The figure shows three views and two pictorial views of one solid part (mm, origin at its lowest corner). Answer the questions. A direction names the side the tool comes from. Round coordinates to 2 decimals unless told otherwise and drop trailing zeros. Write each loop counter-clockwise with the first axis right and the second up, starting at its lowest first coordinate (ties: lowest second). Pieces come first, ordered by that corner, then holes.
Item 1: A tool of negligible diameter and unlimited length cuts with its end or side. For the marked faces 4 and 5, from which of +Z, -Z, +X, -X, +Y, -Y can it reach the whole face along a straight path? Write none if from no direction.
Item 2: Find section D-D on z = 36. Give the vertices of the cut face in (x, y).
Item 3: Find section B-B on z = 23.5. Give the vertices of the cut face in (x, y).
Item 4: For a pull along X with two mould halves and no side action, classify the marked faces 1, 2 and 3 as +X half, -X half, draft (parallel to the pull), parting line (faces both ways), or undercut.
Item 5: Find section A-A on x = 23.5. Give the vertices of the cut face in (y, z).
Item 6: Each of these flat-tipped pins is pushed along its axis until it touches: pin 1 (3 mm diameter, centred on x = 41.5, z = 31.5, fed in from -Y); pin 2 (6 mm diameter, centred on y = 3.5, z = 35.5, fed in from -X); pin 3 (1.5 mm diameter, centred on x = 19, y = 7.5, fed in from +Z); pin 4 (3 mm diameter, centred on x = 39.5, y = 17, fed in from -Z). Where does it stop, or does it pass through?
Item 7: Find section C-C on y = 24.25. Give the number of separate pieces and of enclosed holes in the cut face.
Item 8: Find the intervals of material crossed by probe 1 along X at (y, z) = (9.5, 23.5); probe 2 along Z at (x, y) = (11, 20.75) (1 decimal); probe 3 along X at (y, z) = (20.5, 25.5), in increasing order.
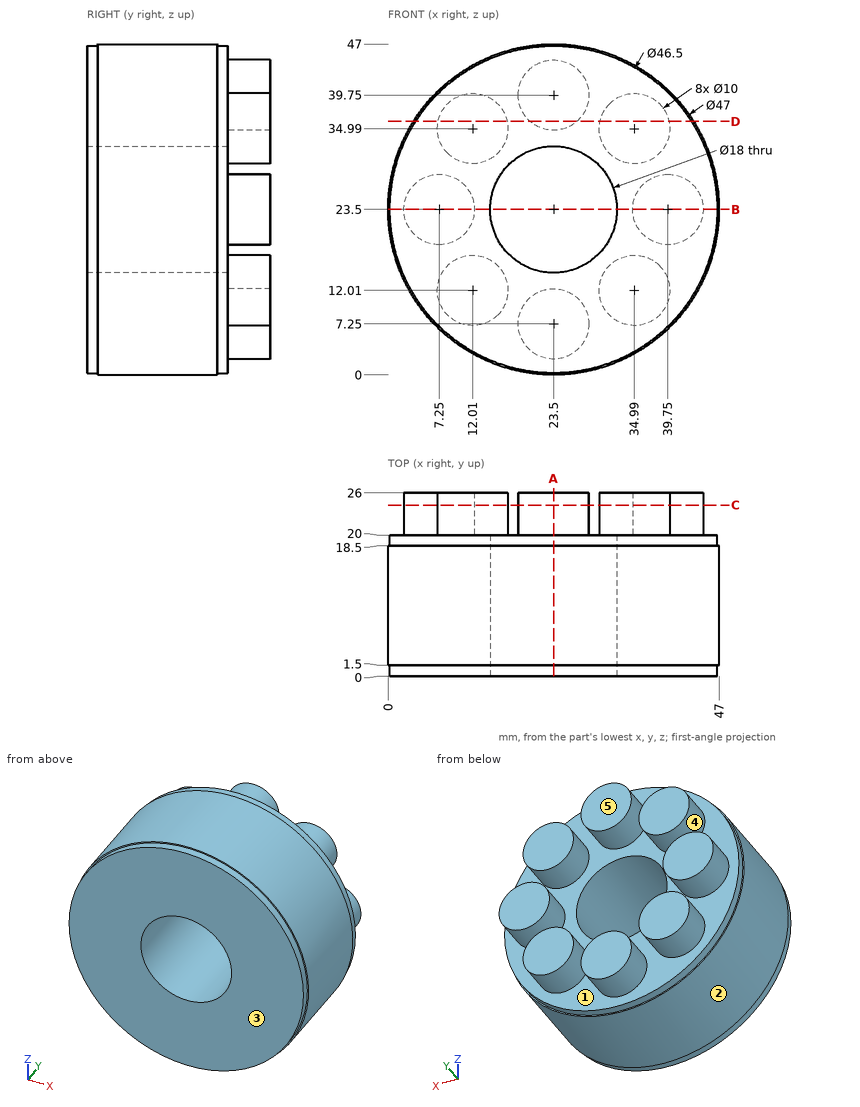
Check values:
1. face 4: +Y
1. face 5: +Z, -Z, +X, -X, +Y
2. outline: (3.6, 1.5) - (3.9, 1.5) - (3.9, 0) - (43.1, 0) - (43.1, 1.5) - (43.4, 1.5) - (43.4, 18.5) - (43.1, 18.5) - (43.1, 20) - (39.89, 20) - (39.89, 26) - (30.09, 26) - (30.09, 20) - (26.81, 20) - (26.81, 26) - (20.19, 26) - (20.19, 20) - (16.91, 20) - (16.91, 26) - (7.11, 26) - (7.11, 20) - (3.9, 20) - (3.9, 18.5) - (3.6, 18.5) - close
3. outline: (0, 1.5) - (0.25, 1.5) - (0.25, 0) - (14.5, 0) - (14.5, 20) - (12.25, 20) - (12.25, 26) - (2.25, 26) - (2.25, 20) - (0.25, 20) - (0.25, 18.5) - (0, 18.5) - close; (32.5, 0) - (46.75, 0) - (46.75, 1.5) - (47, 1.5) - (47, 18.5) - (46.75, 18.5) - (46.75, 20) - (44.75, 20) - (44.75, 26) - (34.75, 26) - (34.75, 20) - (32.5, 20) - close
4. face 1: undercut
4. face 2: parting line
4. face 3: draft
5. outline: (0, 0.25) - (1.5, 0.25) - (1.5, 0) - (18.5, 0) - (18.5, 0.25) - (20, 0.25) - (20, 2.25) - (26, 2.25) - (26, 12.25) - (20, 12.25) - (20, 14.5) - (0, 14.5) - close; (0, 32.5) - (20, 32.5) - (20, 34.75) - (26, 34.75) - (26, 44.75) - (20, 44.75) - (20, 46.75) - (18.5, 46.75) - (18.5, 47) - (1.5, 47) - (1.5, 46.75) - (0, 46.75) - close
6. pin 1: stops at y = 0
6. pin 2: stops at x = 1.79
6. pin 3: stops at z = 46.7
6. pin 4: stops at z = 5.01
7. separate pieces: 8
7. enclosed holes: 0
8. probe 1: x = 0 to 14.5, 32.5 to 47
8. probe 2: z = 7.1 to 16.9, 20.2 to 26.8, 30.1 to 39.9
8. probe 3: x = 2.67 to 11.83, 35.17 to 44.33
